from build123d import *

# Parameters (mm, degrees)
BASE_FLANGE1_DEPTH      = 25.4
CUT_EXTRUDE1_DEPTH      = 62.700339563
CUT_EXTRUDE1_DEPTH_BACK = 62.700339563
SKETCH6_R               = 2.4892
CUT_EXTRUDE4_DEPTH      = 63.904146145
FILLET1_R               = 1.5875


# Sheet-metal steps are written as plain solids
with BuildPart() as part:
    # Sketch1 → Base-Flange1 (new body)
    with BuildSketch(Plane.XY):
        with BuildLine():
            Line((-53.2765, -6.35), (-53.2765, 5.588))
            ThreePointArc((-53.2765, 5.588), (-53.053315367, 6.126815367), (-52.5145, 6.35))
            Line((-52.5145, 6.35), (52.5145, 6.35))
            ThreePointArc((52.5145, 6.35), (53.053315367, 6.126815367), (53.2765, 5.588))
            Line((53.2765, 5.588), (53.2765, -6.35))
            Line((53.2765, -6.35), (55.5625, -6.35))
            Line((55.5625, -6.35), (55.5625, 5.588))
            ThreePointArc((55.5625, 5.588), (54.669761469, 7.743261469), (52.5145, 8.636))
            Line((52.5145, 8.636), (-52.5145, 8.636))
            ThreePointArc((-52.5145, 8.636), (-54.669761469, 7.743261469), (-55.5625, 5.588))
            Line((-55.5625, 5.588), (-55.5625, -6.35))
            Line((-55.5625, -6.35), (-53.2765, -6.35))
        make_face()
    extrude(amount=BASE_FLANGE1_DEPTH)

    # Sketch6 → Cut-Extrude1 (cut, two sides: drawn at the far end of the back side and taken through both)
    with BuildSketch(Plane(origin=(0, 0, 0), x_dir=(0, 0, -1), z_dir=(1, 0, 0)).offset(-CUT_EXTRUDE1_DEPTH_BACK)):
        with Locations((19.05, -0.888959106)):
            Circle(SKETCH6_R)
        with Locations((6.35, -0.888959106)):
            Circle(SKETCH6_R)
        with Locations((-6.35, -0.888959106)):
            Circle(SKETCH6_R)
        with Locations((-19.05, -0.888959106)):
            Circle(SKETCH6_R)
    extrude(amount=CUT_EXTRUDE1_DEPTH + CUT_EXTRUDE1_DEPTH_BACK, mode=Mode.SUBTRACT)

    # Sketch8 → Cut-Extrude4 (cut, through all)
    with BuildSketch(Plane(origin=(0, 8.636, 0), x_dir=(1, 0, 0), z_dir=(0, 1, 0))):
        Polygon((49.3395, -19.152466608), (49.3395, -6.247533392), (38.1635, -12.7), align=None)
        Polygon((49.3395, -22.225), (49.3395, -20.985553713), (37.36975, -14.074815329), (37.36975, -22.225), align=None)
        Polygon((35.78225, -22.225), (35.78225, -14.074815329), (21.665716058, -22.225), align=None)
        Polygon((19.08175, -21.883766394), (34.9885, -12.7), (19.08175, -3.516233606), align=None)
        Polygon((35.78225, -11.325184671), (35.78225, -3.175), (21.665716058, -3.175), align=None)
        Polygon((37.36975, -11.325184671), (49.3395, -4.414446287), (49.3395, -3.175), (37.36975, -3.175), align=None)
        Polygon((17.49425, -21.883766394), (17.49425, -3.516233606), (1.5875, -12.7), align=None)
        Polygon((0.79375, -22.225), (14.910283942, -22.225), (0.79375, -14.074815329), align=None)
        Polygon((0.79375, -11.325184671), (14.910283942, -3.175), (0.79375, -3.175), align=None)
        Polygon((-0.79375, -11.325184671), (-0.79375, -3.175), (-14.910283942, -3.175), align=None)
        Polygon((-17.49425, -21.883766394), (-1.5875, -12.7), (-17.49425, -3.516233606), align=None)
        Polygon((-14.910283942, -22.225), (-0.79375, -22.225), (-0.79375, -14.074815329), align=None)
        Polygon((-19.08175, -21.883766394), (-19.08175, -3.516233606), (-34.9885, -12.7), align=None)
        Polygon((-35.78225, -22.225), (-21.665716058, -22.225), (-35.78225, -14.074815329), align=None)
        Polygon((-35.78225, -11.325184671), (-21.665716058, -3.175), (-35.78225, -3.175), align=None)
        Polygon((-37.36975, -11.325184671), (-37.36975, -3.175), (-49.3395, -3.175), (-49.3395, -4.414446287), align=None)
        Polygon((-49.3395, -19.152466608), (-38.1635, -12.7), (-49.3395, -6.247533392), align=None)
        Polygon((-49.3395, -22.225), (-37.36975, -22.225), (-37.36975, -14.074815329), (-49.3395, -20.985553713), align=None)
    extrude(amount=-CUT_EXTRUDE4_DEPTH, mode=Mode.SUBTRACT)

    # Fillet1
    # the kernel refuses this fillet: 1.5875 mm, written as the material it adds along each edge
    with BuildSketch(Plane(origin=(37.36975, 8.636, 3.175), x_dir=(0, 0, 1), z_dir=(0, -1, 0)), Plane(origin=(49.3395, 8.636, 3.175), x_dir=(-1, 0, 0), z_dir=(0, -1, 0)), Plane(origin=(49.3395, 8.636, 22.225), x_dir=(0, 0, -1), z_dir=(0, -1, 0)), Plane(origin=(35.78225, 8.636, 22.225), x_dir=(0, 0, -1), z_dir=(0, -1, 0)), Plane(origin=(35.78225, 8.636, 3.175), x_dir=(-1, 0, 0), z_dir=(0, -1, 0)), Plane(origin=(-49.3395, 8.636, 3.175), x_dir=(0, 0, 1), z_dir=(0, -1, 0)), Plane(origin=(-37.36975, 8.636, 3.175), x_dir=(-1, 0, 0), z_dir=(0, -1, 0)), Plane(origin=(-0.79375, 8.636, 3.175), x_dir=(-1, 0, 0), z_dir=(0, -1, 0)), Plane(origin=(-0.79375, 8.636, 22.225), x_dir=(0, 0, -1), z_dir=(0, -1, 0)), Plane(origin=(-37.36975, 8.636, 22.225), x_dir=(0, 0, -1), z_dir=(0, -1, 0)), Plane(origin=(-49.3395, 8.636, 22.225), x_dir=(1, 0, 0), z_dir=(0, -1, 0))) as fillet1_piece_1:
        with BuildLine():
            CenterArc((FILLET1_R, -FILLET1_R), FILLET1_R, 90, 90)
            Line((0, -FILLET1_R), (0, 0))
            Line((0, 0), (FILLET1_R, 0))
        make_face()
    extrude(amount=2.286)
    with BuildSketch(Plane(origin=(49.3395, 8.636, 4.414446287), x_dir=(0, 0, -1), z_dir=(0, -1, 0)), Plane(origin=(49.3395, 8.636, 20.985553713), x_dir=(-0.8660254037844429, 0, -0.4999999999999925), z_dir=(0, -1, 0)), Plane(origin=(-49.3395, 8.636, 4.414446287), x_dir=(0.8660254037844405, 0, 0.4999999999999969), z_dir=(0, -1, 0)), Plane(origin=(-49.3395, 8.636, 20.985553713), x_dir=(0, 0, 1), z_dir=(0, -1, 0))) as fillet1_piece_2:
        with BuildLine():
            CenterArc((FILLET1_R * 0.57735026919, -FILLET1_R), FILLET1_R, 90, 60)
            Line((-FILLET1_R * 0.288675134595, -FILLET1_R * 0.5), (0, 0))
            Line((0, 0), (FILLET1_R * 0.57735026919, 0))
        make_face()
    extrude(amount=2.286)
    with BuildSketch(Plane(origin=(37.36975, 8.636, 11.325184671), x_dir=(0, 0, -1), z_dir=(0, -1, 0)), Plane(origin=(1.5875, 8.636, 12.7), x_dir=(0.8660254037844406, 0, -0.4999999999999966), z_dir=(0, -1, 0)), Plane(origin=(35.78225, 8.636, 11.325184671), x_dir=(-0.8660254037844403, 0, -0.49999999999999717), z_dir=(0, -1, 0)), Plane(origin=(19.08175, 8.636, 21.883766394), x_dir=(0, 0, -1), z_dir=(0, -1, 0)), Plane(origin=(-37.36975, 8.636, 11.325184671), x_dir=(-0.8660254037844397, 0, -0.49999999999999817), z_dir=(0, -1, 0)), Plane(origin=(-49.3395, 8.636, 19.152466608), x_dir=(0, 0, -1), z_dir=(0, -1, 0)), Plane(origin=(-17.49425, 8.636, 21.883766394), x_dir=(0, 0, -1), z_dir=(0, -1, 0)), Plane(origin=(-0.79375, 8.636, 11.325184671), x_dir=(-0.8660254037844397, 0, -0.4999999999999983), z_dir=(0, -1, 0)), Plane(origin=(-0.79375, 8.636, 14.074815329), x_dir=(0, 0, 1), z_dir=(0, -1, 0)), Plane(origin=(-34.9885, 8.636, 12.7), x_dir=(0.8660254037844405, 0, -0.49999999999999667), z_dir=(0, -1, 0)), Plane(origin=(-37.36975, 8.636, 14.074815329), x_dir=(0, 0, 1), z_dir=(0, -1, 0)), Plane(origin=(49.3395, 8.636, 19.152466608), x_dir=(-0.8660254037844397, 0, -0.49999999999999817), z_dir=(0, -1, 0))) as fillet1_piece_3:
        with BuildLine():
            CenterArc((FILLET1_R * 1.73205080757, FILLET1_R), FILLET1_R, 150, 120)
            Line((FILLET1_R * 0.866025403784, FILLET1_R * 1.5), (0, 0))
            Line((0, 0), (FILLET1_R * 1.73205080757, 0))
        make_face()
    extrude(amount=2.286)
    with BuildSketch(Plane(origin=(17.49425, 8.636, 3.516233606), x_dir=(-0.8660254037844396, 0, 0.49999999999999817), z_dir=(0, -1, 0)), Plane(origin=(17.49425, 8.636, 21.883766394), x_dir=(0, 0, -1), z_dir=(0, -1, 0)), Plane(origin=(0.79375, 8.636, 14.074815329), x_dir=(0, 0, 1), z_dir=(0, -1, 0)), Plane(origin=(0.79375, 8.636, 11.325184671), x_dir=(0.8660254037844398, 0, -0.4999999999999979), z_dir=(0, -1, 0)), Plane(origin=(37.36975, 8.636, 14.074815329), x_dir=(0, 0, 1), z_dir=(0, -1, 0)), Plane(origin=(35.78225, 8.636, 14.074815329), x_dir=(-0.8660254037844395, 0, 0.4999999999999986), z_dir=(0, -1, 0)), Plane(origin=(19.08175, 8.636, 3.516233606), x_dir=(0, 0, 1), z_dir=(0, -1, 0)), Plane(origin=(34.9885, 8.636, 12.7), x_dir=(-0.866025403784439, 0, -0.4999999999999993), z_dir=(0, -1, 0)), Plane(origin=(-38.1635, 8.636, 12.7), x_dir=(-0.8660254037844394, 0, -0.4999999999999986), z_dir=(0, -1, 0)), Plane(origin=(-49.3395, 8.636, 6.247533392), x_dir=(0, 0, 1), z_dir=(0, -1, 0)), Plane(origin=(-35.78225, 8.636, 11.325184671), x_dir=(0.86602540378444, 0, -0.49999999999999767), z_dir=(0, -1, 0)), Plane(origin=(-35.78225, 8.636, 14.074815329), x_dir=(0, 0, 1), z_dir=(0, -1, 0)), Plane(origin=(-17.49425, 8.636, 3.516233606), x_dir=(0, 0, 1), z_dir=(0, -1, 0)), Plane(origin=(-1.5875, 8.636, 12.7), x_dir=(-0.8660254037844406, 0, -0.4999999999999966), z_dir=(0, -1, 0)), Plane(origin=(-19.08175, 8.636, 3.516233606), x_dir=(-0.8660254037844397, 0, 0.499999999999998), z_dir=(0, -1, 0)), Plane(origin=(-19.08175, 8.636, 21.883766394), x_dir=(0, 0, -1), z_dir=(0, -1, 0)), Plane(origin=(49.3395, 8.636, 6.247533392), x_dir=(-0.8660254037844402, 0, 0.4999999999999975), z_dir=(0, -1, 0)), Plane(origin=(38.1635, 8.636, 12.7), x_dir=(0.8660254037844394, 0, 0.4999999999999986), z_dir=(0, -1, 0))) as fillet1_piece_4:
        with BuildLine():
            CenterArc((FILLET1_R * 1.73205080757, -FILLET1_R), FILLET1_R, 90, 120)
            Line((FILLET1_R * 0.866025403784, -FILLET1_R * 1.5), (0, 0))
            Line((0, 0), (FILLET1_R * 1.73205080757, 0))
        make_face()
    extrude(amount=2.286)
    with BuildSketch(Plane(origin=(14.910283942, 8.636, 22.225), x_dir=(-0.8660254037844399, 0, -0.49999999999999767), z_dir=(0, -1, 0)), Plane(origin=(14.910283942, 8.636, 3.175), x_dir=(-1, 0, 0), z_dir=(0, -1, 0)), Plane(origin=(21.665716058, 8.636, 3.175), x_dir=(0.8660254037844398, 0, 0.4999999999999979), z_dir=(0, -1, 0)), Plane(origin=(-21.665716058, 8.636, 3.175), x_dir=(-1, 0, 0), z_dir=(0, -1, 0)), Plane(origin=(-21.665716058, 8.636, 22.225), x_dir=(-0.8660254037844397, 0, -0.49999999999999806), z_dir=(0, -1, 0)), Plane(origin=(-14.910283942, 8.636, 3.175), x_dir=(0.8660254037844397, 0, 0.499999999999998), z_dir=(0, -1, 0)), Plane(origin=(-14.910283942, 8.636, 22.225), x_dir=(1, 0, 0), z_dir=(0, -1, 0))) as fillet1_piece_5:
        with BuildLine():
            CenterArc((FILLET1_R * 3.73205080757, -FILLET1_R), FILLET1_R, 90, 150)
            Line((FILLET1_R * 3.23205080757, -FILLET1_R * 1.86602540378), (0, 0))
            Line((0, 0), (FILLET1_R * 3.73205080757, 0))
        make_face()
    extrude(amount=2.286)
    with BuildSketch(Plane(origin=(0.79375, 8.636, 22.225), x_dir=(0, 0, -1), z_dir=(0, -1, 0)), Plane(origin=(0.79375, 8.636, 3.175), x_dir=(1, 0, 0), z_dir=(0, -1, 0)), Plane(origin=(37.36975, 8.636, 22.225), x_dir=(0, 0, -1), z_dir=(0, -1, 0)), Plane(origin=(-35.78225, 8.636, 3.175), x_dir=(1, 0, 0), z_dir=(0, -1, 0)), Plane(origin=(-35.78225, 8.636, 22.225), x_dir=(0, 0, -1), z_dir=(0, -1, 0))) as fillet1_piece_6:
        with BuildLine():
            CenterArc((FILLET1_R, FILLET1_R), FILLET1_R, 180, 90)
            Line((0, FILLET1_R), (0, 0))
            Line((0, 0), (FILLET1_R, 0))
        make_face()
    extrude(amount=2.286)
    with BuildSketch(Plane(origin=(21.665716058, 8.636, 22.225), x_dir=(0.8660254037844399, 0, -0.49999999999999784), z_dir=(0, -1, 0))) as fillet1_piece_7:
        with BuildLine():
            CenterArc((FILLET1_R * 3.73205080757, FILLET1_R), FILLET1_R, 120, 150)
            Line((FILLET1_R * 3.23205080757, FILLET1_R * 1.86602540378), (0, 0))
            Line((0, 0), (FILLET1_R * 3.73205080757, 0))
        make_face()
    extrude(amount=2.286)


solid = part.part
Verification items for the finished model (mm, model axes). A direction names the side the tool comes from. Round coordinates to 2 decimals unless told otherwise and drop trailing zeros. Loops run counter-clockwise (first coordinate to the right, second up) from the corner with the lowest first, then second, coordinate; pieces in that order, holes last. Notation, with made-up numbers: M -31.75,22 L 22.25,22 A31 cw 22.25,49 Z; hole C 63,2.5 d7. An arc over 180 degrees is marked long. Write each question's results on one line, items separated by ' | '.
1) Gauge pin test, flat ends, axial feed: P1, Ø2.5, axis at y = 7.5, z = 10.5, coming from the +X side; P2, Ø2, axis at x = 39.5, y = 4, coming from the +Z side; P3, Ø2.5, axis at y = 8, z = 18.5, coming from the +X side; P4, Ø2.5, axis at y = 7.5, z = 19.5, coming from the -X side. Record the tip position at first contact, or that the pin passes through.
Checks:
P1: stops at x = 55.49 | P2: passes through | P3: stops at x = 55.33 | P4: stops at x = -55.49
2) Mould release check, pull along X, two halves, no side actions. Record for faces 1 (the cylindrical face through (1.608, 7.509, 9.962)), 2 (the flat face through (-35.782, 8, 19)), 3 (the cylindrical face through (54.69, 7.72, 12.52)): released by +X, released by -X, zero draft, split by the parting line, or undercut.
Checks:
face 1: undercut | face 2: undercut | face 3: released by +X
3) Section check A-A on y = -5. Record the boundary of the cut face in (x, z), then the cut area to 3 significant figures.
Checks:
outline: M -55.56,0 L -53.28,0 L -53.28,25.4 L -55.56,25.4 Z; M 53.28,0 L 55.56,0 L 55.56,25.4 L 53.28,25.4 Z | area: 116 mm2
4) Access from +Z, -Z, +X, -X, +Y, -Y to the whole of each face (thin tool, end or side, straight path). Record for faces 4 (the flat face through (0, 6.35, 13)), 5 (the flat face through (6.52, 7.51, 17.38)).
Checks:
face 4: +Z, -Z, -Y | face 5: +Y, -Y
5) Section check B-B on x = 6. Record the boundary of the cut face in (y, z) (3 decimals).
Checks:
outline: M 6.35,0 L 8.636,0 L 8.636,3.175 L 6.35,3.175 Z; M 6.35,8.319 L 8.636,8.319 L 8.636,10.152 L 6.35,10.152 Z; M 6.35,15.248 L 8.636,15.248 L 8.636,17.081 L 6.35,17.081 Z; M 6.35,22.225 L 8.636,22.225 L 8.636,25.4 L 6.35,25.4 Z
6) Scan lines: L1, parallel to Z at x = -7.5, y = 7 (3 decimals); L2, parallel to X at y = 5.75, z = 11; L3, parallel to Z at x = -27.5, y = 7.5. Record each from-to range of solid material in increasing order. Write a range as from..to.
Checks:
L1: z = 0..3.175, 7.453..9.286, 16.114..17.947, 22.225..25.4 | L2: x = -55.56..-53.26, 53.26..55.56 | L3: z = 0..3.18, 6.54..8.38, 17.02..18.86, 22.22..25.4
